Could you check a few things on this model? Use its own coordinates, in mm. Face numbers are marked on the shaded views. A direction names the side the tool comes from. Coordinates: 2 decimals unless noted, no trailing zeros. Loops run counter-clockwise (first coordinate to the right, second up) from the corner with the lowest first, then second, coordinate; pieces in that order, holes last.
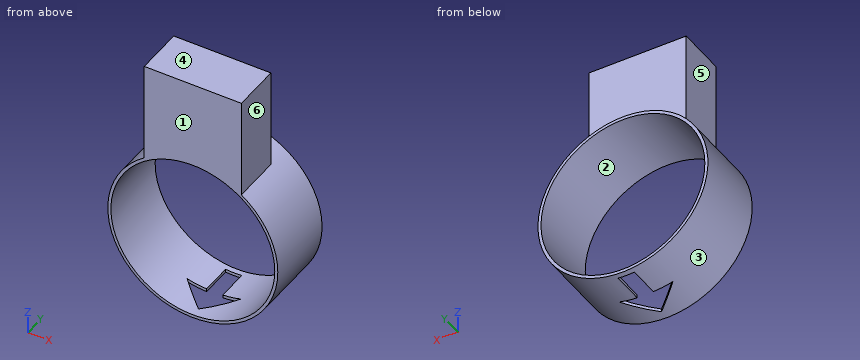
from build123d import *

# Parameters (mm, degrees)
F0_R     = 88.9
F1_DEPTH = 76.2
F2_W     = 101.6
F2_H     = 50.8
F3_DEPTH = 177.8
F5_DEPTH = 304.8
F6_R     = 85.725
F7_DEPTH = 76.201


with BuildPart() as f1:
    # F0 (on Front) → F1 (new body)
    with BuildSketch(Plane.XZ):
        Circle(F0_R)
    extrude(amount=F1_DEPTH)

    # F2 (on Top) → F3 (join)
    with BuildSketch(Plane.XY):
        with Locations((0, -50.8)):
            Rectangle(F2_W, F2_H)
    extrude(amount=F3_DEPTH)

    # F4 (on Top) → F5 (cut)
    with BuildSketch(Plane.XY):
        Polygon((8.465788, -5.836729), (0, -5.836729), (-8.465788, -5.836729), (-8.465788, -38.511038), (-28.219294, -39.673008), (0, -66.438295), (28.219294, -39.673008), (8.465788, -38.511038), align=None)
    extrude(amount=-F5_DEPTH, mode=Mode.SUBTRACT)

    # F6 (on face) → F7 (cut, through all)
    with BuildSketch(Plane.XZ.offset(76.2)):
        Circle(F6_R)
    extrude(amount=-F7_DEPTH, mode=Mode.SUBTRACT)


solid = f1.part
(1) Which directions (+Z, -Z, +X, -X, +Y, -Y) give clear straight access to the entire face, cutting with the end or side of a thin tool? Please do the marked faces 4, 5 and 6.
Answers:
face 4: +Z, +X, -X, +Y, -Y
face 5: +Z, -X, +Y, -Y
face 6: +Z, +X, +Y, -Y
(2) We'd pull the mould along X, two halves only. Please class the marked faces 1, 2 and 3: +X half, -X half, draft (parallel to the pull), parting line (faces both ways), or undercut.
Answers:
face 1: draft
face 2: undercut
face 3: parting line
(3) Imagine slicing it at B-B, the plane x = -24. Write out the boundary of the cut face in (y, z), and give its area (3 significant figures).
Answers:
outline: (-76.2, -85.6) - (-43.67, -85.6) - (-43.67, -82.3) - (-76.2, -82.3) - close; (-76.2, 82.3) - (0, 82.3) - (0, 85.6) - (-25.4, 85.6) - (-25.4, 177.8) - (-76.2, 177.8) - close; (-39.42, -85.6) - (0, -85.6) - (0, -82.3) - (-39.42, -82.3) - close
area: 5,170 mm2
(4) I need wall thicknesses on probe 1 along Z at (x, y) = (0, -43.5) (3 decimals); probe 2 along X at (y, z) = (-66, 134); probe 3 along Z at (x, y) = (34, -69). Which ranges of each line are inside material? Lowest first, please.
Answers:
probe 1: z = 85.725 to 177.8
probe 2: x = -50.8 to 50.8
probe 3: z = -82.14 to -78.69, 78.69 to 177.8
(5) Imagine slicing it at A-A, the plane z = -58. Write out the boundary of the cut face in (x, y).
Answers:
outline: (-67.37, -76.2) - (-63.13, -76.2) - (-63.13, 0) - (-67.37, 0) - close; (63.13, -76.2) - (67.37, -76.2) - (67.37, 0) - (63.13, 0) - close
(6) For pin 1 (1 mm diameter, centred on y = -15.5, z = 44, fed in from +X); pin 2 (15 mm diameter, centred on y = -62.5, z = 112.5, fed in from +X); pin 3 (5 mm diameter, centred on x = -17.5, z = 115.5, fed in from +Y); pin 4 (5 mm diameter, centred on y = -13.5, z = 2, fed in from -X), each with a flat end and sliding along its axis, tell me the tip position at first contact or that it passes through.
Answers:
pin 1: stops at x = 77.53
pin 2: stops at x = 50.8
pin 3: stops at y = -25.4
pin 4: stops at x = -88.9
(7) Imagine slicing it at C-C, the plane y = -71. Write out the boundary of the cut face in (x, z) (3 decimals), and give its area (3 significant figures).
Answers:
outline: (-50.8, 72.956) arc R88.9 ccw (long way) to (50.8, 72.956) - (50.8, 177.8) - (-50.8, 177.8) - close; hole circle Ø171.45 at (0, 0)
area: 11,300 mm2
(8) Imagine slicing it at D-D, the plane x = 42. Write out the boundary of the cut face in (y, z).
Answers:
outline: (-76.2, -78.35) - (0, -78.35) - (0, -74.73) - (-76.2, -74.73) - close; (-76.2, 74.73) - (0, 74.73) - (0, 78.35) - (-25.4, 78.35) - (-25.4, 177.8) - (-76.2, 177.8) - close
